Input: part model. Units: mm. Frame: model coordinates. Face numbers are marked on the shaded views. A direction names the side the tool comes from. Coordinates: 2 decimals unless noted, no trailing zeros. Loops run counter-clockwise (first coordinate to the right, second up) from the corner with the lowest first, then second, coordinate; pieces in that order, holes last.
Item 1: Pull-direction query (Y, two-part tool) for the marked faces 1, 2, 3 and 4; classes: released by +Y, released by -Y, zero draft, split by the parting line, or undercut.
Item 2: Ray query, line 1 along Z through (x, y) = (-6.25, -1.5) (3 decimals); line 2 along X through (y, z) = (3, 2.5); line 3 along Y through (x, z) = (1.5, 3.25) (3 decimals). Return the intervals inside material, ascending.
Item 3: Section D-D on z = 12.5. Return loops of the section in (x, y) (3 decimals), and give its area (3 significant figures).
Item 4: Section B-B on z = 5. Return loops of the section in (x, y) (3 decimals).
Item 5: Reachability of the marked faces 5, 6 and 7 from +Z, -Z, +X, -X, +Y, -Y: full face, straight path, thin tool, end or side. Return the list, or none.
Item 6: Section A-A on x = 0. Return loops of the section in (y, z) (3 decimals).
Item 7: Contact query for flat-ended pins moving along their axis: P1, Ø1, axis at x = 7, y = -6, coming from the -Z side; P2, Ø3.5, axis at x = 6.5, y = 4.5, coming from the +Z side (3 decimals); P3, Ø1, axis at x = -2, z = 2, coming from the +Y side; P4, Ø5, axis at y = 3.5, z = 11.5, coming from the -X side. Output: stop coordinate, or through.
Item 8: Section C-C on y = -2.5. Return loops of the section in (x, z) (3 decimals), and give its area (3 significant figures).
```python
from build123d import *

# Parameters (mm, degrees)
SKETCH1_R           = 9.5
BOSS_EXTRUDE1_DEPTH = 14.185
SKETCH2_R           = 3.5
CUT_EXTRUDE1_DEPTH  = 2


with BuildPart() as part:
    # Sketch1 → Boss-Extrude1 (new body)
    with BuildSketch(Plane.XY):
        with Locations(Location((0, 0, 0), (0, 0, 180))):
            Circle(SKETCH1_R)
        Polygon((1.890822132, -3.275), (-1.890822132, -3.275), (-3.781644263, 0), (-1.890822132, 3.275), (1.890822132, 3.275), (3.781644263, 0), align=None, mode=Mode.SUBTRACT)
    extrude(amount=BOSS_EXTRUDE1_DEPTH)

    # Sketch2 → Cut-Extrude1 (cut)
    with BuildSketch(Plane.XY.offset(14.185)):
        with Locations((5.499261314, 3.175)):
            Circle(SKETCH2_R)
        with Locations((-5.499261314, -3.175)):
            Circle(SKETCH2_R)
    extrude(amount=-CUT_EXTRUDE1_DEPTH, mode=Mode.SUBTRACT)


solid = part.part
```
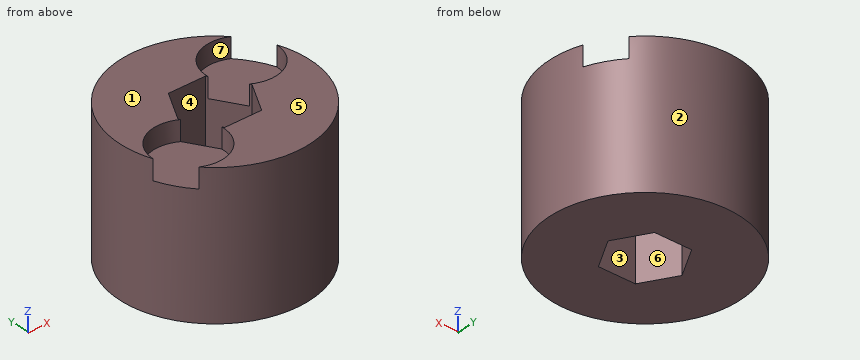
Results found:
1. face 1: zero draft
1. face 2: split by the parting line
1. face 3: undercut
1. face 4: undercut
2. line 1: z = 0 to 12.185
2. line 2: x = -9.01 to -2.05, 2.05 to 9.01
2. line 3: y = -9.381 to -3.275, 3.275 to 9.381
3. outline: (-8.997, -3.05) arc R3.5 cw to (-3.672, -0.19) - (-3.782, 0) - (-1.891, 3.275) - (1.891, 3.275) - (2, 3.085) arc R3.5 cw to (7.14, 6.267) arc R9.5 ccw to start; (-7.14, -6.267) arc R9.5 ccw to (8.997, 3.05) arc R3.5 cw to (3.672, 0.19) - (3.782, 0) - (1.891, -3.275) - (-1.891, -3.275) - (-2, -3.085) arc R3.5 cw to start
3. area: 173 mm2
4. outline: circle Ø19 at (0, 0); hole (-3.782, 0) - (-1.891, -3.275) - (1.891, -3.275) - (3.782, 0) - (1.891, 3.275) - (-1.891, 3.275) - close
5. face 5: +Z, +X, -X, +Y, -Y
5. face 6: +Z, -Z
5. face 7: +Z
6. outline: (-9.5, 0) - (-3.275, 0) - (-3.275, 14.185) - (-9.5, 14.185) - close; (3.275, 0) - (9.5, 0) - (9.5, 14.185) - (3.275, 14.185) - close
7. P1: stops at z = 0
7. P2: stops at z = 12.185
7. P3: stops at y = 9.38
7. P4: stops at x = -9.45
8. outline: (-9.165, 0) - (-2.338, 0) - (-2.338, 12.185) - (-8.934, 12.185) - (-8.934, 14.185) - (-9.165, 14.185) - close; (2.338, 0) - (9.165, 0) - (9.165, 14.185) - (2.338, 14.185) - close
8. area: 180 mm2
